The listing builds one solid part. Answer for the finished solid, in the listing's coordinates (mm). Round coordinates to 2 decimals unless told otherwise and drop trailing zeros. Use a Markdown table: item, result. Add a question column.
1) A cutting plane is placed at A-A (z = 1.05). State how many separate pieces and enclosed holes the cut face has, then the cut area to 3 significant figures.
2) Find the intervals of material crossed by probe 1 along Y at (x, z) = (0, 1.95); probe 2 along X at (y, z) = (1.75, 3.8); probe 3 along X at (y, z) = (2.75, 3.15), in increasing order. Write a range as from..to.
3) This flat-tipped pin is pushed along its axis until it touches: P1, Ø2.5, axis at y = 2.5, z = 1.5, coming from the -X side. Where does it stop, or does it pass through?
```python
from build123d import *

# Parameters (mm, degrees)
SKETCH_1_R          = 1.5
EXTRUDE_1_DEPTH     = 5
SKETCH_3_W          = 5
SKETCH_3_H          = 10
CUT_EXTRUDE_1_DEPTH = 351.258832865


with BuildPart() as part:
    # 스케치1 → 보스-돌출1 (new body)
    with BuildSketch(Plane.XY):
        with BuildLine():
            Line((0, -12.5), (350, -12.5))
            Line((350, -12.5), (350, -5))
            Line((350, -5), (345, -5))
            Line((345, -5), (345, 5))
            Line((345, 5), (350, 5))
            Line((350, 5), (350, 12.5))
            Line((350, 12.5), (0, 12.5))
            ThreePointArc((0, 12.5), (-12.5, 0), (0, -12.5))
        make_face()
        with Locations((7.116257118, 0)):
            Circle(SKETCH_1_R, mode=Mode.SUBTRACT)
        with Locations((-7.116257118, 0)):
            Circle(SKETCH_1_R, mode=Mode.SUBTRACT)
        with Locations((0, 7.25)):
            Circle(SKETCH_1_R, mode=Mode.SUBTRACT)
        with Locations((0, -7.25)):
            Circle(SKETCH_1_R, mode=Mode.SUBTRACT)
    extrude(amount=EXTRUDE_1_DEPTH)

    # 스케치3 → 컷-돌출1 (cut, through all)
    with BuildSketch(Plane(origin=(0, 0, 0), x_dir=(-1, 0, 0), z_dir=(0, 0, -1))):
        with Locations((-272.5, 0)):
            Rectangle(SKETCH_3_W, SKETCH_3_H)
        with Locations((-192.5, 0)):
            Rectangle(SKETCH_3_W, SKETCH_3_H)
        with Locations((-132.5, 0)):
            Rectangle(SKETCH_3_W, SKETCH_3_H)
        with Locations((-62.5, 0)):
            Rectangle(SKETCH_3_W, SKETCH_3_H)
    extrude(amount=-CUT_EXTRUDE_1_DEPTH, mode=Mode.SUBTRACT)


solid = part.part
```
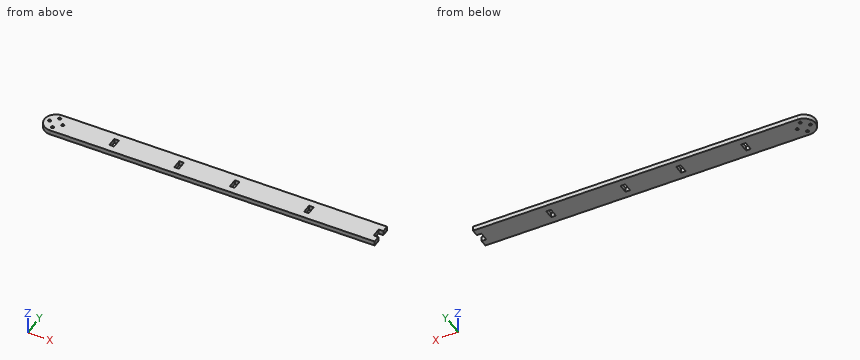
Entries:
| question | item | result |
|---|---|---|
| 1 | separate pieces | 1 |
| 1 | enclosed holes | 8 |
| 1 | area | 8,720 mm² |
| 2 | probe 1 | y = -12.5..-8.75, -5.75..5.75, 8.75..12.5 |
| 2 | probe 2 | x = -12.38..60, 65..130, 135..190, 195..270, 275..345 |
| 2 | probe 3 | x = -12.19..60, 65..130, 135..190, 195..270, 275..345 |
| 3 | P1 | stops at x = -12.44 |
